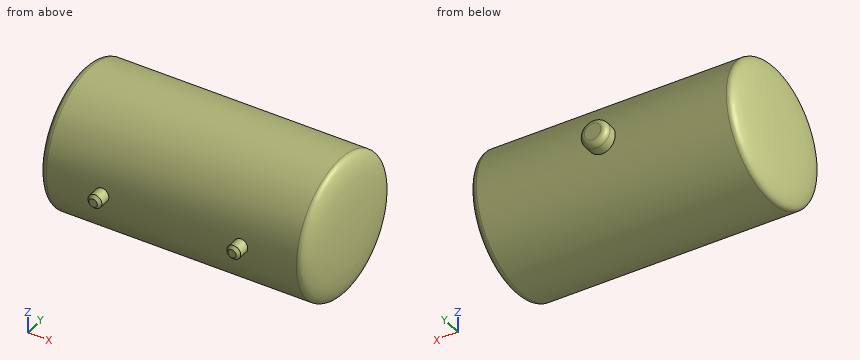
from build123d import *

# Parameters (mm, degrees)
SKETCH1_R           = 25
BOSS_EXTRUDE1_DEPTH = 45
SKETCH3_R           = 5
BOSS_EXTRUDE2_DEPTH = 30
FILLET1_R           = 2
SKETCH4_R           = 2.5
BOSS_EXTRUDE3_DEPTH = 30
CHAMFER1_SIZE       = 1


with BuildPart() as part:
    # Sketch1 → Boss-Extrude1 (new, symmetric)
    with BuildSketch(Plane(origin=(0, 0, 0), x_dir=(0, 0, -1), z_dir=(1, 0, 0))):
        with Locations(Location((0, 0, 0), (0, 0, 180))):
            Circle(SKETCH1_R)
    extrude(amount=BOSS_EXTRUDE1_DEPTH, both=True)

    # Sketch2 → Revolve1 (revolve)
    with BuildSketch(Plane.XY):
        with BuildLine():
            Line((-45, 25), (-45, 0))
            Line((-45, 0), (-50, 0))
            add(Edge.make_bspline(
                [(-45, 25), (-50, 25), (-50, 0)],
                knots=[0, 0, 0, 1, 1, 1], degree=2))
        make_face()
    revolve(axis=Axis((-45, 0, 0), (-1, 0, 0)))

    # Sketch2_4 → Revolve2 (revolve)
    with BuildSketch(Plane.XY):
        with BuildLine():
            add(Edge.make_bspline(
                [(45, 25), (50, 25), (50, 0)],
                knots=[0, 0, 0, 1, 1, 1], degree=2))
            Line((50, 0), (45, 0))
            Line((45, 0), (45, 25))
        make_face()
    revolve(axis=Axis((45, 0, 0), (1, 0, 0)))

    # Sketch3 → Boss-Extrude2 (add)
    with BuildSketch(Plane(origin=(0, 0, 0), x_dir=(1, 0, 0), z_dir=(0, 1, 0))):
        with Locations(Location((0, 0, 0), (0, 0, 90))):
            Circle(SKETCH3_R)
    extrude(amount=BOSS_EXTRUDE2_DEPTH)

    # Fillet1
    fillet1_edges = [part.edges().sort_by_distance(p)[0] for p in [
        (0, 30, 5),
    ]]
    fillet(fillet1_edges, radius=FILLET1_R)

    # Sketch4 → Boss-Extrude3 (add)
    with BuildSketch(Plane(origin=(0, 0, 0), x_dir=(1, 0, 0), z_dir=(0, 1, 0))):
        with Locations(Location((-25, 0, 0), (0, 0, 270))):
            Circle(SKETCH4_R)
        with Locations(Location((25, 0, 0), (0, 0, 270))):
            Circle(SKETCH4_R)
    extrude(amount=-BOSS_EXTRUDE3_DEPTH)

    # Chamfer1
    chamfer1_edges = [part.edges().sort_by_distance(p)[0] for p in [
        (-25, -30, -2.5),
        (25, -30, -2.5),
    ]]
    chamfer(chamfer1_edges, length=CHAMFER1_SIZE)


solid = part.part
Verification items for the finished model (mm, model axes). Coordinates: 2 decimals unless noted, no trailing zeros. Order: outer loops, then holes, each group sorted by start corner. A loop starts at its lowest first (then second) coordinate and runs counter-clockwise, first axis right, second up.
1. Sectioned sample at A-A, the plane x = 25. Record the cut outline in (y, z).
Results found:
outline: (-30, -1.5) - (-29, -2.5) - (-24.87, -2.5) arc R25 ccw (long way) to (-24.87, 2.5) - (-29, 2.5) - (-30, 1.5) - close
2. Scan lines: line 1 (Z direction, x = 25, y = 1); line 2 (Y direction, x = 41, z = 4); line 3 (X direction, y = -4, z = -23). Record each from-to range of solid material in increasing order.
Results found:
line 1: z = -24.98 to 24.98
line 2: y = -24.68 to 24.68
line 3: x = -47.24 to 47.24
3. Go/stop test with flat-tipped pins: pin 1 Ø3 at (y, z) = (2, -5.5) entering from -X; pin 2 Ø1.5 at (x, z) = (-28.5, -10) entering from +Y; pin 3 Ø4 at (x, z) = (23, 14.5) entering from +Y. Record where each tip stops, or that it passes through.
Results found:
pin 1: stops at x = -49.96
pin 2: stops at y = 23.23
pin 3: stops at y = 21.65
4. Sectioned sample at B-B, the plane x = 0. Record the cut outline in (y, z).
Results found:
outline: (24.49, -5) - (28, -5) arc R2 ccw to (30, -3) - (30, 3) arc R2 ccw to (28, 5) - (24.49, 5) arc R25 ccw (long way) to start
5. Sectioned sample at C-C, the plane x = 11. Record the cut outline in (y, z).
Results found:
outline: circle Ø50 at (0, 0)
